from build123d import *

# Parameters (mm, degrees)
BOSS_EXTRUDE1_DEPTH = 5


with BuildPart() as part:
    # Sketch1 → Boss-Extrude1 (new body)
    with BuildSketch(Plane.XY):
        with BuildLine():
            Line((-5, 13.882591105), (-5, 8.902615006))
            Line((-5, 8.902615006), (-5, 4))
            Line((-5, 4), (0, 4))
            Line((0, 4), (0, 0))
            Line((0, 0), (-251.584289061, 0))
            Line((-251.584289061, 0), (-251.584289061, 32.048381087))
            Line((-251.584289061, 32.048381087), (-82.810223158, 32.048381087))
            ThreePointArc((-82.810223158, 32.048381087), (-80.060223158, 34.798381087), (-82.810223158, 37.548381087))
            Line((-82.810223158, 37.548381087), (-251.584289061, 37.548381087))
            Line((-251.584289061, 37.548381087), (-251.584289061, 86.350886134))
            Line((-251.584289061, 86.350886134), (0, 86.350886134))
            Line((0, 86.350886134), (0, 68.247704672))
            Line((0, 68.247704672), (-5, 68.247704672))
            Line((-5, 68.247704672), (-5, 48.006517598))
            Line((-5, 48.006517598), (-22, 48.006517598))
            Line((-22, 48.006517598), (-22, 22.779366172))
            Line((-22, 22.779366172), (-5, 22.779366172))
            Line((-5, 22.779366172), (-5, 13.882591105))
        make_face()
    extrude(amount=-BOSS_EXTRUDE1_DEPTH)


solid = part.part
Here's how the part is built. I have some questions about the finished solid (model axes, mm). A direction names the side the tool comes from. Give positions to 0.01 mm unless a question says otherwise; leave off trailing zeros. Order: outer loops, then holes, each group sorted by start corner. A loop starts at its lowest first (then second) coordinate and runs counter-clockwise, first axis right, second up. Notation, with made-up numbers: (41.5, 79.25) -> (59.5, 79.25) arc R31 ccw to (59.5, 118.25) -> close; hole circle Ø9 at (-14, -9.75). An arc over 180 degrees is marked (long way). Use a Markdown table: item, result. Add a question column.
Item 1: Will these pins go through, and if not, where does the flat tip stop? pin 1 (4 mm diameter, centred on x = -66.5, y = 35.5, fed in from +Z); pin 2 (2.5 mm diameter, centred on y = 34.5, z = -2, fed in from +X); pin 3 (2.5 mm diameter, centred on y = 58, z = -3.5, fed in from +X).
Item 2: Imagine slicing it at C-C on y = 13. Please give me the cut outline in (x, z).
Item 3: I need wall thicknesses on line 1 (Y direction, x = -87.5, z = -1.45); line 2 (X direction, y = 47, z = -3.35); line 3 (X direction, y = 50.5, z = -4.1). Which ranges of each line are inside material? Lowest first, please.
Item 4: For faces 4 (the face through (-168, 32.048, -2)), 5 (the face through (-13, 48.007, -2)), 6 (the face through (0, 77, -2)), which set-ups out of +Z, -Z, +X, -X, +Y, -Y let a thin tool reach every point of the face, with its end or its side?
Item 5: If we mould it in two halves opening along Y, with no side actions, what happens to faces 1 (the face through (-5, 14, -2)), 2 (the face through (-251.584, 16, -2)), 3 (the face through (-124, 0, -2))? For each: pulls with the +Y half, pulls with the -Y half, needs draft (parallel to the pull), parting line crosses it, or undercut.
Item 6: Imagine slicing it at B-B on z = -3.35. Please give me the cut outline in (x, y).
Item 7: Imagine slicing it at A-A on x = -175. Please give me the cut outline in (y, z).
Data:
| question | item | result |
|---|---|---|
| 1 | pin 1 | stops at z = 0 |
| 1 | pin 2 | stops at x = -22 |
| 1 | pin 3 | stops at x = -5 |
| 2 | outline | (-251.58, -5) -> (-5, -5) -> (-5, 0) -> (-251.58, 0) -> close |
| 3 | line 1 | y = 0 to 32.05, 37.55 to 86.35 |
| 3 | line 2 | x = -251.58 to -22 |
| 3 | line 3 | x = -251.58 to -5 |
| 4 | face 4 | +Z, -Z, -X |
| 4 | face 5 | +Z, -Z, +X |
| 4 | face 6 | +Z, -Z, +X, +Y, -Y |
| 5 | face 1 | undercut |
| 5 | face 2 | needs draft |
| 5 | face 3 | pulls with the -Y half |
| 6 | outline | (-251.58, 0) -> (0, 0) -> (0, 4) -> (-5, 4) -> (-5, 22.78) -> (-22, 22.78) -> (-22, 48.01) -> (-5, 48.01) -> (-5, 68.25) -> (0, 68.25) -> (0, 86.35) -> (-251.58, 86.35) -> (-251.58, 37.55) -> (-82.81, 37.55) arc R2.75 cw to (-82.81, 32.05) -> (-251.58, 32.05) -> close |
| 7 | outline | (0, -5) -> (32.05, -5) -> (32.05, 0) -> (0, 0) -> close; (37.55, -5) -> (86.35, -5) -> (86.35, 0) -> (37.55, 0) -> close |
